Verification items for the finished model (mm, model axes). A direction names the side the tool comes from. Give positions to 0.01 mm unless a question says otherwise; leave off trailing zeros. Order: outer loops, then holes, each group sorted by start corner. A loop starts at its lowest first (then second) coordinate and runs counter-clockwise, first axis right, second up. Notation, with made-up numbers: (40, 43) -> (57, 43) arc R10 cw to (57, 52) -> close; hole circle Ø6 at (-24, 79). An arc over 180 degrees is marked (long way). One line per question, with ' | ' between items. Start each with the question number.
Q1. Section check A-A on z = 0. Record the cut outline in (x, y), plus the area to 3 significant figures.
Q2. Section check C-C on x = -42. Record the cut outline in (y, z).
Q3. Access from +Z, -Z, +X, -X, +Y, -Y to the whole of each face (thin tool, end or side, straight path). Record for faces 1 (the cylindrical face through (-0.28, -30.04, 95.38)), 2 (the flat face through (20, -24, 43)), 3 (the cylindrical face through (-33.94, -14.51, 46.08)).
Q4. Section check D-D on y = 32. Record the cut outline in (x, z), plus the area to 3 significant figures.
Q5. Material ranges on probe 1 along X at (y, z) = (-83, 21.5); probe 2 along Z at (x, y) = (19.5, -1) (3 decimals); probe 3 along Y at (x, z) = (-41, -14), recorded low to high. Write a range as [from, to].
Q6. Go/stop test with flat-tipped pins: pin 1 (1 mm diameter, centred on y = -65.5, z = 68.5, fed in from -X); pin 2 (1 mm diameter, centred on y = 52.5, z = 26, fed in from +X); pin 3 (6 mm diameter, centred on x = -5.5, y = 13.5, fed in from -Z). Record where each tip stops, or that it passes through.
from build123d import *


with BuildPart() as part:
    # 草图1 → 旋转1 (revolve)
    with BuildSketch(Plane.XY, mode=Mode.PRIVATE) as revolve_1_sk:
        Polygon((0, 0), (0, 100), (20, 100), (20, 48.308684326), (47.5, 48.308684326), (47.5, 6), (85, 6), (85, 0), align=None)
    revolve_1 = revolve(revolve_1_sk.sketch.rotate(Axis((-1219.943710548, 0, 0), (1, 0, 0)), 90), axis=Axis((-1219.943710548, 0, 0), (1, 0, 0)))

    # 镜向1: 旋转1 across plane
    add(revolve_1.mirror(Plane(origin=(0, 0, 0), x_dir=(0, 0, 1), z_dir=(1, 0, 0))))


solid = part.part
Filled in:
1) outline: (-85, -6) -> (-47.5, -6) -> (-47.5, -48.31) -> (-20, -48.31) -> (-20, -100) -> (20, -100) -> (20, -48.31) -> (47.5, -48.31) -> (47.5, -6) -> (85, -6) -> (85, 6) -> (47.5, 6) -> (47.5, 48.31) -> (20, 48.31) -> (20, 100) -> (-20, 100) -> (-20, 48.31) -> (-47.5, 48.31) -> (-47.5, 6) -> (-85, 6) -> close | area: 14,200 mm²
2) outline: circle Ø96.62 at (0, 0)
3) face 1: +X, -X | face 2: +X | face 3: -X
4) outline: (-47.5, -36.19) -> (-20, -36.19) -> (-20, -94.74) -> (20, -94.74) -> (20, -36.19) -> (47.5, -36.19) -> (47.5, 36.19) -> (20, 36.19) -> (20, 94.74) -> (-20, 94.74) -> (-20, 36.19) -> (-47.5, 36.19) -> close | area: 11,600 mm²
5) probe 1: [-20, 20] | probe 2: [-99.995, 99.995] | probe 3: [-46.24, 46.24]
6) pin 1: x = -20 | pin 2: x = 20 | pin 3: z = -99.45
